```python
from build123d import *

# Parameters (mm, degrees)
F0_R      = 3.25
F0_R_2    = 2.25
F1_DEPTH  = 100
F0_R_3    = 5
F2_DEPTH  = 95
F0_R_4    = 7.5
F3_DEPTH  = 5
F4_DEPTH  = 20
F6_R      = 5.5
F7_DEPTH  = 2
F8_R      = 2
F9_DEPTH  = 12.5
F10_R     = 2
F11_DEPTH = 12.5


# Not quite as in the source:
# - a fillet or chamfer that OpenCascade refuses, or shapes differently, is made with other operations: its cross-section is extruded or revolved along the edge and cut away or added


with BuildPart() as f1:
    # F0 (on Top) → F1 (new body)
    with BuildSketch(Plane.XY):
        Circle(F0_R)
        Circle(F0_R_2, mode=Mode.SUBTRACT)
    extrude(amount=F1_DEPTH)

    # F0 (on Top) → F2 (join)
    with BuildSketch(Plane.XY):
        Circle(F0_R_3)
        Circle(F0_R, mode=Mode.SUBTRACT)
    extrude(amount=F2_DEPTH)

    # F0 (on Top) → F3 (join)
    with BuildSketch(Plane.XY):
        Circle(F0_R_4)
        Circle(F0_R_3, mode=Mode.SUBTRACT)
    extrude(amount=F3_DEPTH)

    # F0 (on Top) → F4 (join)
    with BuildSketch(Plane.XY):
        Circle(F0_R_4)
        Circle(F0_R_3, mode=Mode.SUBTRACT)
    extrude(amount=-F4_DEPTH)

    # F6 (on offset) → F7 (join)
    with BuildSketch(Plane(origin=(0, 0, -20), x_dir=(1, 0, 0), z_dir=(0, 0, -1))):
        Circle(F6_R)
    extrude(amount=-F7_DEPTH)

    # F8 (on Front) → F9 (cut, symmetric)
    with BuildSketch(Plane.XZ):
        with Locations((0, -13)):
            Circle(F8_R)
    extrude(amount=F9_DEPTH, both=True, mode=Mode.SUBTRACT)

    # F10 (on Right) → F11 (cut, symmetric)
    with BuildSketch(Plane.YZ):
        with Locations((0, -14)):
            Circle(F10_R)
    extrude(amount=F11_DEPTH, both=True, mode=Mode.SUBTRACT)

    # F12: fillet of radius 3 on 1 edges, made by hand

    # F12_s1 → F12_t2 (revolve, cut)
    with BuildSketch(Plane.XZ):
        with BuildLine():
            ThreePointArc((5, 5), (6.7912878475, 3.9784517816), (7.5, 2.0419601084))
            Line((7.5, 2.0419601084), (7.5, 5))
            Line((7.5, 5), (5, 5))
        make_face()
    revolve(axis=Axis((0, 0, 5), (0, 0, 1)), mode=Mode.SUBTRACT)


solid = f1.part
```
Geometry: final body of the model. Coordinates: model frame, mm. A direction names the side the tool comes from. Round coordinates to 2 decimals unless told otherwise and drop trailing zeros. Loops run counter-clockwise (first coordinate to the right, second up) from the corner with the lowest first, then second, coordinate; pieces in that order, holes last. Notation, with made-up numbers: (88, 42) -> (106, 42) arc R31 cw to (106, 72) -> close; hole circle Ø11 at (41, 83.25). An arc over 180 degrees is marked (long way). Use one line per item in the form item = value.
Item 1: Cut plane A-A on y = 0. Output: boundary loops of the cut face in (x, z), then the cut area to 3 significant figures.
Evaluation:
outline = (-7.5, -20) -> (7.5, -20) -> (7.5, -16) -> (5, -16) -> (5, -18) -> (-5, -18) -> (-5, -16) -> (-7.5, -16) -> close; (-7.5, -12) -> (-5, -12) -> (-5, 0) -> (-2.25, 0) -> (-2.25, 100) -> (-3.25, 100) -> (-3.25, 95) -> (-5, 95) -> (-5, 5) arc R3 ccw to (-7.5, 2.04) -> close; (2.25, 0) -> (5, 0) -> (5, -12) -> (7.5, -12) -> (7.5, 2.04) arc R3 ccw to (5, 5) -> (5, 95) -> (3.25, 95) -> (3.25, 100) -> (2.25, 100) -> close
area = 654 mm2
Item 2: Access query for faces 4 (the flat face through (0, 0, -20)), 5 (the cylindrical face through (2.307, -4.436, -8.874)), 6 (the cylindrical face through (-0.29, 2.23, 49.3)). Directions: +Z, -Z, +X, -X, +Y, -Y. A direction counts if a zero-diameter tool reaches every point of the face in a straight line with its end or side. Return the directions, or none.
Evaluation:
face_4 = -Z, +X, -X, +Y, -Y
face_5 = none
face_6 = +Z
Item 3: Draft query along X for faces 1 (the flat face through (2.2, -1, 0)), 2 (the cylindrical face through (-2.579, -1.978, 97.465)), 3 (the flat face through (1, -3.3, 95)). Return one class per face: released by +X, released by -X, zero draft, split by the parting line, or undercut.
Evaluation:
face_1 = undercut
face_2 = split by the parting line
face_3 = zero draft
Item 4: Cut plane B-B on x = 0. Output: boundary loops of the cut face in (y, z), then the cut area to 3 significant figures.
Evaluation:
outline = (-7.5, -20) -> (7.5, -20) -> (7.5, -15) -> (5, -15) -> (5, -18) -> (-5, -18) -> (-5, -15) -> (-7.5, -15) -> close; (-7.5, -11) -> (-5, -11) -> (-5, 0) -> (-2.25, 0) -> (-2.25, 100) -> (-3.25, 100) -> (-3.25, 95) -> (-5, 95) -> (-5, 5) arc R3 ccw to (-7.5, 2.04) -> close; (2.25, 0) -> (5, 0) -> (5, -11) -> (7.5, -11) -> (7.5, 2.04) arc R3 ccw to (5, 5) -> (5, 95) -> (3.25, 95) -> (3.25, 100) -> (2.25, 100) -> close
area = 654 mm2
Item 5: Cut plane D-D on z = -13. Output: boundary loops of the cut face in (x, y), then the cut area to 3 significant figures.
Evaluation:
outline = (-7.3, -1.73) arc R7.5 ccw to (-2, -7.23) -> (-2, -4.58) arc R5 cw to (-4.69, -1.73) -> close; (-7.3, 1.73) -> (-4.69, 1.73) arc R5 cw to (-2, 4.58) -> (-2, 7.23) arc R7.5 ccw to start; (2, -7.23) arc R7.5 ccw to (7.3, -1.73) -> (4.69, -1.73) arc R5 cw to (2, -4.58) -> close; (2, 4.58) arc R5 cw to (4.69, 1.73) -> (7.3, 1.73) arc R7.5 ccw to (2, 7.23) -> close
area = 60.2 mm2
Item 6: Material intervals for probe 1 along Z at (x, y) = (-0.25, 3.5); probe 2 along Y at (x, z) = (0, -4.5); probe 3 along X at (y, z) = (5.6, -13), sorted ascending.
Evaluation:
probe_1 = -20 to -18, 0 to 95
probe_2 = -7.5 to -5, 5 to 7.5
probe_3 = -4.99 to -2, 2 to 4.99
Item 7: Cut plane C-C on z = 76. Output: boundary loops of the cut face in (x, y), then the cut area to 3 significant figures.
Evaluation:
outline = circle Ø10 at (0, 0); hole circle Ø4.5 at (0, 0)
area = 62.6 mm2
Item 8: Contact query for flat-ended pins moving along their axis: pin 1 Ø3.5 at (x, y) = (0, 0) entering from +Z; pin 2 Ø1.5 at (y, z) = (4, 67.5) entering from -X; pin 3 Ø5 at (x, y) = (6, 3) entering from +Z. Output: stop coordinate, or through.
Evaluation:
pin_1 = -18
pin_2 = -3.8
pin_3 = 95
